from build123d import *

# Parameters (mm, degrees)
CROQUIS1_W              = 22
CROQUIS1_H              = 4
SALIENTE_EXTRUIR1_DEPTH = 3
CROQUIS2_R              = 0.85
CORTAR_EXTRUIR1_DEPTH   = 3
CORTAR_EXTRUIR2_REACH   = 13.576
CROQUIS3_R              = 1


with BuildPart() as part:
    # Croquis1 → Saliente-Extruir1 (new body)
    with BuildSketch(Plane.XY):
        Rectangle(CROQUIS1_W, CROQUIS1_H)
    extrude(amount=SALIENTE_EXTRUIR1_DEPTH)

    # Croquis2 → Cortar-Extruir1 (cut)
    with BuildSketch(Plane(origin=(0, 2, 0), x_dir=(1, 0, 0), z_dir=(0, 1, 0))):
        with Locations(Location((-1, -1.5, 0), (0, 0, 270))):
            Circle(CROQUIS2_R)
    extrude(amount=-CORTAR_EXTRUIR1_DEPTH, mode=Mode.SUBTRACT)

    # Croquis3 → Cortar-Extruir2 (cut, up to next)
    with BuildSketch(Plane.XY.offset(3), mode=Mode.PRIVATE) as cortar_extruir2_sk1:
        with Locations((8.5, -0.5)):
            Circle(CROQUIS3_R)
    cortar_extruir2_tool1 = extrude(cortar_extruir2_sk1.sketch, amount=-CORTAR_EXTRUIR2_REACH, mode=Mode.PRIVATE) & part.part
    # Croquis3 → Cortar-Extruir2 (cut, up to next)
    with BuildSketch(Plane.XY.offset(3), mode=Mode.PRIVATE) as cortar_extruir2_sk2:
        with Locations((-9.5, 0)):
            Circle(CROQUIS3_R)
    cortar_extruir2_tool2 = extrude(cortar_extruir2_sk2.sketch, amount=-CORTAR_EXTRUIR2_REACH, mode=Mode.PRIVATE) & part.part
    add(cortar_extruir2_tool1.solids().sort_by_distance((8.5, -0.5, 3))[0], mode=Mode.SUBTRACT)
    add(cortar_extruir2_tool2.solids().sort_by_distance((-9.5, 0, 3))[0], mode=Mode.SUBTRACT)


solid = part.part
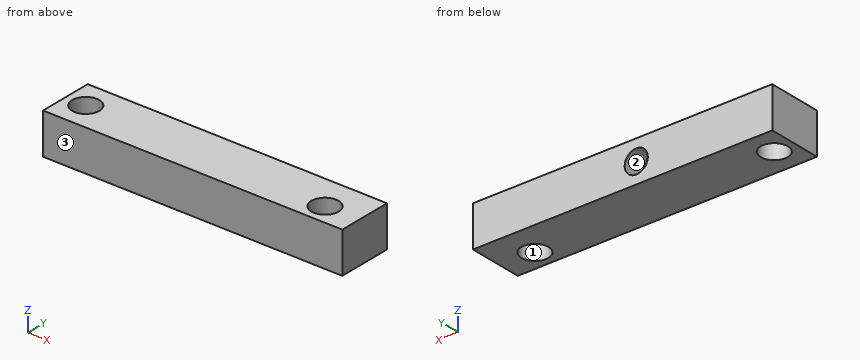
Here's how the part is built. I have some questions about the finished solid (model axes, mm). Face numbers are marked on the shaded views. Round coordinates to 2 decimals unless told otherwise and drop trailing zeros. Order: outer loops, then holes, each group sorted by start corner. A loop starts at its lowest first (then second) coordinate and runs counter-clockwise, first axis right, second up. Notation, with made-up numbers: (15, 61) -> (26, 61) arc R34 ccw to (26, 98) -> close; hole circle Ø1 at (11, 48.5). An arc over 180 degrees is marked (long way). Return JSON: item names as keys, results as strings.
Q1. I need wall thicknesses on line 1 along Y through (x, z) = (8.5, 1); line 2 along Y through (x, z) = (-9.5, 0.6); line 3 along X through (y, z) = (0.15, 1.3). Which ranges of each line are inside material? Lowest first, please. Write a range as from..to.
Filled sheet:
{"line 1": "y = -2..-1.5, 0.5..2", "line 2": "y = -2..-1, 1..2", "line 3": "x = -11..-10.49, -8.51..-1.83, -0.17..7.74, 9.26..11"}
Q2. If we section it at B-B on x = -9.5: List the corners of the cut face in (y, z) for me, plus the area to 3 significant figures.
Filled sheet:
{"outline": "(-2, 0) -> (-1, 0) -> (-1, 3) -> (-2, 3) -> close; (1, 0) -> (2, 0) -> (2, 3) -> (1, 3) -> close", "area": "6.00 mm^2"}
Q3. If we section it at C-C on z = 1.1: List the corners of the cut face in (x, y) for me, plus the area to 3 significant figures.
Filled sheet:
{"outline": "(-11, -2) -> (11, -2) -> (11, 2) -> (-0.25, 2) -> (-0.25, -1) -> (-1.75, -1) -> (-1.75, 2) -> (-11, 2) -> close; hole circle Ø2 at (-9.5, 0); hole circle Ø2 at (8.5, -0.5)", "area": "77.2 mm^2"}
Q4. For pin 1 Ø1.2 at (x, y) = (8.5, -0.5) entering from +Z; pin 2 Ø1.5 at (x, z) = (-1, 1.5) entering from +Y, each with a flat end and sliding along its axis, tell me the tip position at first contact or that it passes through.
Filled sheet:
{"pin 1": "passes through", "pin 2": "stops at y = -1"}
Q5. If we mould it in two halves opening along Y, with no side actions, what happens to the marked faces 1, 2 and 3? For each: released by +Y, released by -Y, zero draft, split by the parting line, or undercut.
Filled sheet:
{"face 1": "undercut", "face 2": "zero draft", "face 3": "released by -Y"}
Q6. If we section it at D-D on x = -1: List the corners of the cut face in (y, z) for me, plus the area to 3 significant figures.
Filled sheet:
{"outline": "(-2, 0) -> (2, 0) -> (2, 0.65) -> (-1, 0.65) -> (-1, 2.35) -> (2, 2.35) -> (2, 3) -> (-2, 3) -> close", "area": "6.90 mm^2"}
Q7. If we section it at A-A on y = 0: List the corners of the cut face in (x, z) for me.
Filled sheet:
{"outline": "(-11, 0) -> (-10.5, 0) -> (-10.5, 3) -> (-11, 3) -> close; (-8.5, 0) -> (7.63, 0) -> (7.63, 3) -> (-8.5, 3) -> close; (9.37, 0) -> (11, 0) -> (11, 3) -> (9.37, 3) -> close; hole circle Ø1.7 at (-1, 1.5)"}
